Check sheet for the modelled part. Datum: model origin and axes. Units: mm. A direction names the side the tool comes from. Round coordinates to 2 decimals unless told otherwise and drop trailing zeros. Write each loop counter-clockwise with the first axis right and the second up, starting at its lowest first coordinate (ties: lowest second). Pieces come first, ordered by that corner, then holes.
from build123d import *

# Parameters (mm, degrees)
F0_W      = 470
F0_H      = 400
F0_W_2    = 60
F0_H_2    = 20
F1_DEPTH  = 80
F2_W      = 989.0920937061
F2_H      = 720
F3_DEPTH  = 80
F4_R      = 10
F5_DEPTH  = 25
F7_START  = -10
F6_R      = 15
F7_DEPTH  = 40
F10_DEPTH = 80
F12_DEPTH = 890
F13_R     = 5
F15_DEPTH = 1000
F17_DEPTH = 890


with BuildPart() as f1:
    # F0 (on Front) → F1 (new body)
    with BuildSketch(Plane.XZ):
        Polygon((-235, 0), (-355, 0), (-465, 0), (-465, -20), (-355, -20), (-355, -262.1796250343), (-455, -262.1796250343), (-421.8337520964, -312.1796250343), (-355, -312.1796250343), (-355, -1020), (-355, -1040), (-235, -1040), (-235, -840), (235, -840), (235, -1040), (355, -1040), (355, -1020), (355, -240), (410.27864045, -240), (455, -200), (355, -200), (355, -20), (465, -20), (465, 0), (355, 0), (235, 0), (235, -200), (-235, -200), align=None)
        with Locations((0, -520)):
            Rectangle(F0_W, F0_H, mode=Mode.SUBTRACT)
        with Locations((-385, -1030)):
            Rectangle(F0_W_2, F0_H_2)
        with Locations((385, -1030)):
            Rectangle(F0_W_2, F0_H_2)
    extrude(amount=F1_DEPTH)

    # F2 (on face) → F3 (cut)
    with BuildSketch(Plane.XZ.offset(80)):
        with Locations((42.8487956524, -680)):
            Rectangle(F2_W, F2_H)
    extrude(amount=-F3_DEPTH, mode=Mode.SUBTRACT)

    # F4 (on face) → F5 (cut)
    with BuildSketch(Plane.XY):
        with Locations((-400, -40)):
            Circle(F4_R)
        with Locations((400, -40)):
            Circle(F4_R)
    extrude(amount=-F5_DEPTH, mode=Mode.SUBTRACT)

    # F6 (on face) → F7 (join)
    with BuildSketch(Plane.XZ.offset(80).offset(F7_START)):
        with BuildLine():
            Line((-355, -262.1796250343), (-360.3855265494, -221.3018058192))
            ThreePointArc((-360.3855265494, -221.3018058192), (-407.0948116692, -182.2284096551), (-449.9677594515, -225.4765073318))
            Line((-449.9677594515, -225.4765073318), (-455, -262.1796250343))
            Line((-455, -262.1796250343), (-355, -262.1796250343))
        make_face()
        with Locations((-405, -227.1796250343)):
            Circle(F6_R, mode=Mode.SUBTRACT)
        with BuildLine():
            Line((355, -200), (455, -200))
            Line((455, -200), (449.6144734506, -159.1221807849))
            ThreePointArc((449.6144734506, -159.1221807849), (408.6794577223, -120.1506790367), (361.9400684353, -151.9293346135))
            Line((361.9400684353, -151.9293346135), (355, -200))
        make_face()
        with Locations((405, -165)):
            Circle(F6_R, mode=Mode.SUBTRACT)
    extrude(amount=-F7_DEPTH)

    # F9 (on face) → F10 (join)
    with BuildSketch(Plane.XZ.offset(80)):
        Polygon((445, -320), (-445, -320), (-445, -380), (-445, -1040), (-325, -1040), (-325, -380), (325, -380), (325, -1040), (445, -1040), (445, -380), align=None)
    extrude(amount=-F10_DEPTH)

    # F11 (on face) → F12 (cut)
    with BuildSketch(Plane(origin=(-445, 0, 0), x_dir=(0, -1, 0), z_dir=(-1, 0, 0))):
        with BuildLine():
            Line((70, -325), (10, -325))
            ThreePointArc((10, -325), (6.4644660941, -326.4644660941), (5, -330))
            Line((5, -330), (5, -370))
            ThreePointArc((5, -370), (6.4644660941, -373.5355339059), (10, -375))
            Line((10, -375), (70, -375))
            ThreePointArc((70, -375), (73.5355339059, -373.5355339059), (75, -370))
            Line((75, -370), (75, -330))
            ThreePointArc((75, -330), (73.5355339059, -326.4644660941), (70, -325))
        make_face()
    extrude(amount=-F12_DEPTH, mode=Mode.SUBTRACT)

    # F13
    f13_edges = [f1.edges().sort_by_distance(p)[0] for p in [
        (-400, -80, -320),
        (-400, 0, -320),
        (0, -80, -380),
        (0, 0, -380),
        (400, -80, -320),
        (400, 0, -320),
    ]]
    fillet(f13_edges, radius=F13_R)

    # F14 (on face) → F15 (cut)
    with BuildSketch(Plane(origin=(-445, 0, 0), x_dir=(0, -1, 0), z_dir=(-1, 0, 0))):
        Polygon((75, -380), (80, -380), (80, -375), align=None)
        Polygon((0, -375), (0, -380), (5, -380), align=None)
    extrude(amount=-F15_DEPTH, mode=Mode.SUBTRACT)

    # F16 (on face) → F17 (cut)
    with BuildSketch(Plane(origin=(-445, 0, 0), x_dir=(0, -1, 0), z_dir=(-1, 0, 0))):
        with BuildLine():
            ThreePointArc((75, -320), (78.5355339059, -321.4644660941), (80, -325))
            Line((80, -325), (80, -320))
            Line((80, -320), (75, -320))
        make_face()
        with BuildLine():
            ThreePointArc((0, -325), (1.4644660941, -321.4644660941), (5, -320))
            Line((5, -320), (0, -320))
            Line((0, -320), (0, -325))
        make_face()
    extrude(amount=-F17_DEPTH, mode=Mode.SUBTRACT)


solid = f1.part
1. Sectioned sample at C-C, the plane x = 44.5. Enter the section's corners in (y, z), plus the area to 3 significant figures.
2. Go/stop test with flat-tipped pins: pin 1 (2.5 mm diameter, centred on x = 401.5, y = -1.5, fed in from +Z); pin 2 (3 mm diameter, centred on y = -42, z = -796, fed in from +X); pin 3 (12 mm diameter, centred on x = -116.5, y = -37.5, fed in from -Z); pin 4 (2 mm diameter, centred on y = -39.5, z = -650.5, fed in from -X). Record where each tip stops, or that it passes through.
3. Sectioned sample at B-B, the plane z = -472. Enter the section's corners in (x, y), plus the area to 3 significant figures.
4. Set-up check for faces 1 (the flat face through (-452.45, -50.28, -243.57)), 2 (the flat face through (445, -41, -685)), 3 (the flat face through (415, -30, -177)), 4 (the flat face through (-395, -70, -239)), 5 (the flat face through (432.326, -39.44, -220.28)): record each of +Z, -Z, +X, -X, +Y, -Y from which the full face is reachable in a straight line by a thin tool's end or side.
5. Scan lines: line 1 along Z through (x, y) = (277.5, -50); line 2 along X through (y, z) = (-58.5, -601.5); line 3 along X through (y, z) = (-35.5, -82). Record each from-to range of solid material in increasing order.
6. Sectioned sample at A-A, the plane x = -311. Enter the section's corners in (y, z), plus the area to 3 significant figures.
7. Sectioned sample at D-D, the plane z = -342.5. Enter the section's corners in (x, y).
8. Release check for a two-part mould opening along Z. For faces 6 (the cylindrical face through (-390.693, -50.28, -222.674)), 7 (the flat face through (-7, -80, -229)), 8 (the flat face through (-5, -40, -380)) record: released by +Z, released by -Z, zero draft, split by the parting line, or undercut.
Computed values:
1. outline: (-80, -375) - (-75, -380) - (-5, -380) - (0, -375) - (0, -325) arc R5 ccw to (-5, -320) - (0, -320) - (0, -200) - (-80, -200) - (-80, -320) - (-75, -320) arc R5 ccw to (-80, -325) - close; hole (-75, -370) arc R5 ccw to (-70, -375) - (-10, -375) arc R5 ccw to (-5, -370) - (-5, -330) arc R5 ccw to (-10, -325) - (-70, -325) arc R5 ccw to (-75, -330) - close
1. area: 10,900 mm2
2. pin 1: stops at z = 0
2. pin 2: stops at x = 445
2. pin 3: stops at z = -380
2. pin 4: stops at x = -445
3. outline: (-445, -80) - (-325, -80) - (-325, 0) - (-445, 0) - close; (325, -80) - (445, -80) - (445, 0) - (325, 0) - close
3. area: 19,200 mm2
4. face 1: -X, +Y, -Y
4. face 2: -Z, +X, +Y, -Y
4. face 3: +X, +Y
4. face 4: -X, -Y
4. face 5: +X, +Y, -Y
5. line 1: z = -380 to -375, -325 to 0
5. line 2: x = -445 to -325, 325 to 445
5. line 3: x = -355 to -235, 235 to 355
6. outline: (-80, -375) - (-75, -380) - (-5, -380) - (0, -375) - (0, -325) arc R5 ccw to (-5, -320) - (0, -320) - (0, 0) - (-80, 0) - (-80, -320) - (-75, -320) arc R5 ccw to (-80, -325) - close; hole (-75, -370) arc R5 ccw to (-70, -375) - (-10, -375) arc R5 ccw to (-5, -370) - (-5, -330) arc R5 ccw to (-10, -325) - (-70, -325) arc R5 ccw to (-75, -330) - close
6. area: 26,900 mm2
7. outline: (-445, -80) - (445, -80) - (445, -75) - (-445, -75) - close; (-445, -5) - (445, -5) - (445, 0) - (-445, 0) - close
8. face 6: undercut
8. face 7: zero draft
8. face 8: released by -Z
